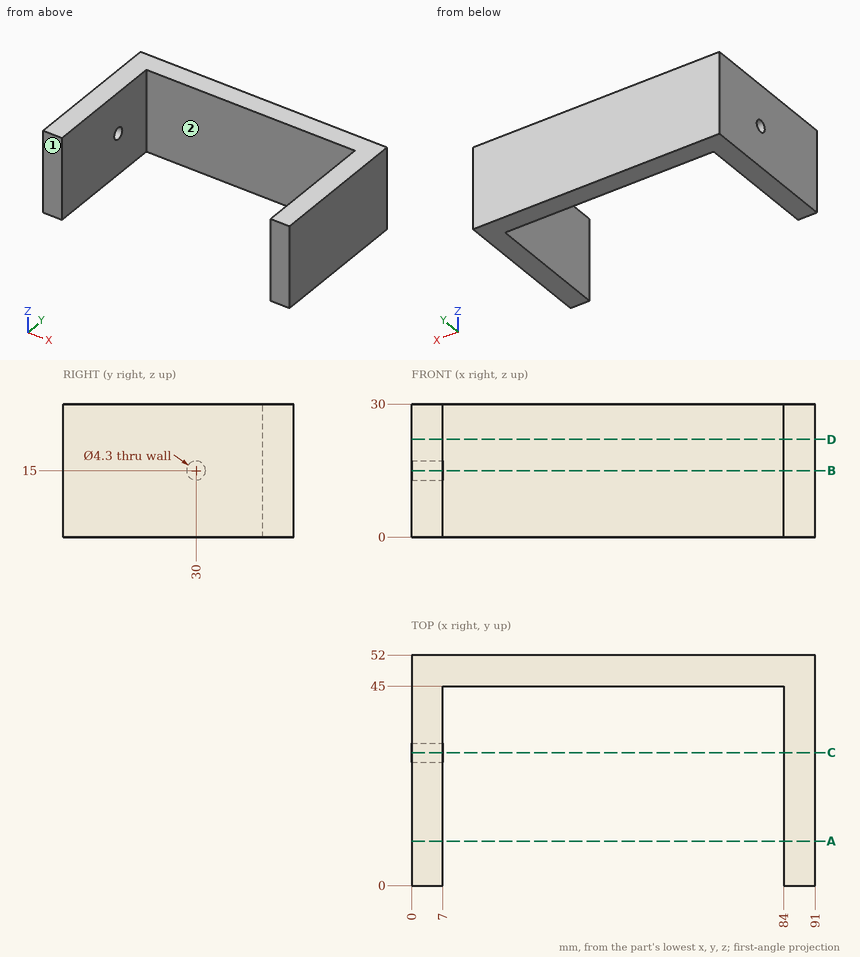
Design review of the part shown in the three views and the two pictorial views. Dimensions are in mm from the part's minimum x, y and z. A direction names the side the tool comes from. Round coordinates to 2 decimals unless told otherwise and drop trailing zeros. Order: outer loops, then holes, each group sorted by start corner. A loop starts at its lowest first (then second) coordinate and runs counter-clockwise, first axis right, second up.
Q1. Wall thickness on line 1 (Z direction, x = 4.75, y = 30); line 2 (X direction, y = 29, z = 12); line 3 (Y direction, x = 83, z = 14.75): over which ranges is each line inside the solid? List them lowest first.
Findings below:
line 1: z = 0 to 12.85, 17.15 to 30
line 2: x = 0 to 7, 84 to 91
line 3: y = 45 to 52
Q2. We need section C-C, the plane y = 30. Give the boundary of the cut face in (x, z), plus the area to 3 significant figures.
Findings below:
outline: (0, 0) - (7, 0) - (7, 12.85) - (0, 12.85) - close; (0, 17.15) - (7, 17.15) - (7, 30) - (0, 30) - close; (84, 0) - (91, 0) - (91, 30) - (84, 30) - close
area: 390 mm2
Q3. We need section D-D, the plane z = 22. Give the boundary of the cut face in (x, y).
Findings below:
outline: (0, 0) - (7, 0) - (7, 45) - (84, 45) - (84, 0) - (91, 0) - (91, 52) - (0, 52) - close
Q4. Machinability: for the marked faces 1 and 2, which of the approach directions +Z, -Z, +X, -X, +Y, -Y give a long, thin tool a straight path to every point of the face, cutting with its end or side? Answer none if there is none.
Findings below:
face 1: +Z, -Z, +X, -X, -Y
face 2: +Z, -Z, -Y
Q5. We need section B-B, the plane z = 15. Give the boundary of the cut face in (x, y), plus the area to 3 significant figures.
Findings below:
outline: (0, 0) - (7, 0) - (7, 27.85) - (0, 27.85) - close; (0, 32.15) - (7, 32.15) - (7, 45) - (84, 45) - (84, 0) - (91, 0) - (91, 52) - (0, 52) - close
area: 1,240 mm2
Q6. Insertion check: P1, Ø15, axis at y = 28.5, z = 21.5, coming from the -X side; P2, Ø8, axis at x = 34, z = 22.5, coming from the -Y side; P3, Ø6, axis at x = 80.5, y = 34.5, coming from the +Z side. Each pin has a flat end and moves straight along its axis. Give the tip position at first contact, or say it passes through.
Findings below:
P1: stops at x = 0
P2: stops at y = 45
P3: passes through
Q7. We need section A-A, the plane y = 10. Give the boundary of the cut face in (x, z), plus the area to 3 significant figures.
Findings below:
outline: (0, 0) - (7, 0) - (7, 30) - (0, 30) - close; (84, 0) - (91, 0) - (91, 30) - (84, 30) - close
area: 420 mm2
